Read the model definition and answer for the solid it produces. Units are mm, in the model's axes. A direction names the side the tool comes from. Give positions to 0.01 mm unless a question says otherwise; leave off trailing zeros. Loops run counter-clockwise (first coordinate to the right, second up) from the corner with the lowest first, then second, coordinate; pieces in that order, holes last. Notation, with made-up numbers: (67, 43.25) - (125, 43.25) arc R15 ccw to (125, 64.25) - close; hole circle Ø5 at (18, 53.5). An arc over 180 degrees is marked (long way). Use a Markdown table: item, result. Add a question column.
Item 1: For a pull along Z with two mould halves and no side action, classify faces 3 (the face through (-3, -200, -3)), 4 (the face through (-3, -2, 188)), 5 (the face through (-2, 4, 106)), 6 (the face through (-3, 3, 190)) as +Z half, -Z half, draft (parallel to the pull), parting line (faces both ways), or undercut.
Item 2: A cutting plane is placed at A-A (z = -19). Determine the outline of the cut face in (x, y), plus the area to 3 significant figures.
Item 3: Consider probe 1 along Z at (x, y) = (89, 19.5); probe 2 along X at (y, z) = (-59, 46). Determine where each line is inside the solid, lowest interval first. Write a range as [from, to].
Item 4: A cutting plane is placed at C-C (y = 85). Determine the outline of the cut face in (x, z).
Item 5: Which of the six approach directions +Z, -Z, +X, -X, +Y, -Y give full straight-line access (tool end or side, diameter ignored) to faces 1 (the face through (-200, 3, 3)), 2 (the face through (198, -44, 178))?
Item 6: A cutting plane is placed at B-B (x = 127). Determine the outline of the cut face in (y, z), plus the area to 3 significant figures.
Item 7: This flat-tipped pin is pushed along its axis until it touches: P1, Ø6, axis at y = 82, z = 74.5, coming from the +X side. Where does it stop, or does it pass through?
from build123d import *

# Parameters (mm, degrees)
SKETCH1_W           = 400
SKETCH1_H           = 380
BOSS_EXTRUDE1_DEPTH = 200
FILLET1_R           = 2
SHELL1_START        = -198
SHELL1_OUTLINE_W    = 398
SHELL1_OUTLINE_H    = 376
SHELL1_DEPTH        = 396
SKETCH2_W           = 350
SKETCH2_H           = 330
CUT_EXTRUDE1_DEPTH  = 485.256130576
BOSS_EXTRUDE2_REACH = 487.901
SKETCH3_W           = 400
SKETCH3_H           = 2


# Read off the part's stored shape, not the designer's step: Shell1
with BuildPart() as part:
    # Sketch1 → Boss-Extrude1 (new, symmetric)
    with BuildSketch(Plane(origin=(0, 0, 0), x_dir=(1, 0, 0), z_dir=(0, 1, 0))):
        Rectangle(SKETCH1_W, SKETCH1_H)
    extrude(amount=BOSS_EXTRUDE1_DEPTH, both=True)

    # Fillet1
    fillet1_edges = [part.edges().sort_by_distance(p)[0] for p in [
        (200, 0, 190),
        (-200, 0, 190),
        (-200, 0, -190),
        (200, 0, -190),
    ]]
    fillet(fillet1_edges, radius=FILLET1_R)

    # Shell1 outline → Shell1 (cut)
    with BuildSketch(Plane.YZ.offset(SHELL1_START)):
        with Locations((1, 0)):
            Rectangle(SHELL1_OUTLINE_W, SHELL1_OUTLINE_H)
    extrude(amount=SHELL1_DEPTH, mode=Mode.SUBTRACT)

    # Sketch2 → Cut-Extrude1 (cut, through all)
    with BuildSketch(Plane.ZY.offset(-198)):
        with Locations((0, 15)):
            Rectangle(SKETCH2_W, SKETCH2_H)
    extrude(amount=-CUT_EXTRUDE1_DEPTH, mode=Mode.SUBTRACT)

    # Sketch3 → Boss-Extrude2 (add, up to next)
    with BuildSketch(Plane(origin=(0, 200, 0), x_dir=(1, 0, 0), z_dir=(0, 1, 0)), mode=Mode.PRIVATE) as boss_extrude2_sk1:
        with Locations((0, -107)):
            Rectangle(SKETCH3_W, SKETCH3_H)
    boss_extrude2_tool1 = extrude(boss_extrude2_sk1.sketch, amount=-BOSS_EXTRUDE2_REACH, mode=Mode.PRIVATE) - part.part
    add(boss_extrude2_tool1.solids().sort_by_distance((0, 200, 107))[0])


solid = part.part
Geometry says:
| question | item | result |
|---|---|---|
| 1 | face 3 | draft |
| 1 | face 4 | undercut |
| 1 | face 5 | undercut |
| 1 | face 6 | +Z half |
| 2 | outline | (-200, -200) - (200, -200) - (200, -150) - (198, -150) - (198, -198) - (-198, -198) - (-198, 200) - (-200, 200) - close; (198, 180) - (200, 180) - (200, 200) - (198, 200) - close |
| 2 | area | 1,730 mm² |
| 3 | probe 1 | [-190, -188], [106, 108], [188, 190] |
| 3 | probe 2 | [-200, -198] |
| 4 | outline | (-200, -188) arc R2 ccw to (-198, -190) - (198, -190) arc R2 ccw to (200, -188) - (200, -175) - (198, -175) - (198, -188) - (-198, -188) - (-198, 106) - (200, 106) - (200, 108) - (-198, 108) - (-198, 188) - (198, 188) - (198, 175) - (200, 175) - (200, 188) arc R2 ccw to (198, 190) - (-198, 190) arc R2 ccw to (-200, 188) - close |
| 5 | face 1 | +Z, -Z, -X, +Y, -Y |
| 5 | face 2 | +Y |
| 6 | outline | (-200, -190) - (200, -190) - (200, -188) - (-198, -188) - (-198, 106) - (200, 106) - (200, 108) - (-198, 108) - (-198, 188) - (200, 188) - (200, 190) - (-200, 190) - close |
| 6 | area | 3,150 mm² |
| 7 | P1 | x = -198 |
